For this review, take the finished solid that the model builds, in its own axes (mm). A direction names the side the tool comes from. Coordinates: 2 decimals unless noted, no trailing zeros. Loops run counter-clockwise (first coordinate to the right, second up) from the corner with the lowest first, then second, coordinate; pieces in that order, holes last. Notation, with made-up numbers: M -12.75,47 L 43.25,47 A16 cw 43.25,77 Z; hole C 2,49.25 d10. An arc over 180 degrees is marked long. Put each result on its own line as item: value.
```python
from build123d import *

# Parameters (mm, degrees)
F0_W     = 220
F0_H     = 25
F0_R     = 5
F1_DEPTH = 25
F2_DEPTH = 25


with BuildPart() as f1:
    # F0 (on Front) → F1 (new body)
    with BuildSketch(Plane.XZ):
        with Locations((103.33334, 12.5)):
            Rectangle(F0_W, F0_H)
        with Locations((3.33334, 12.5)):
            Circle(F0_R, mode=Mode.SUBTRACT)
        with Locations((203.33334, 12.5)):
            Circle(F0_R, mode=Mode.SUBTRACT)
        with Locations((3.33334, 12.5)):
            Circle(F0_R)
        with Locations((203.33334, 12.5)):
            Circle(F0_R)
    extrude(amount=F1_DEPTH)

    # F0 (on Front) → F2 (join)
    with BuildSketch(Plane.XZ):
        with Locations((3.33334, 12.5)):
            Circle(F0_R)
        with Locations((203.33334, 12.5)):
            Circle(F0_R)
    extrude(amount=-F2_DEPTH)


solid = f1.part
```
(1) Add section B-B (y = 12.5). Write out the cut boundary in (x, z).
Determined:
outline: C 3.33,12.5 d10; C 203.33,12.5 d10
(2) Draft analysis for pull direction X (two halves, no side actions). For faces 1 (the flat face through (213.333, -12, 12)), 2 (the cylindrical face through (198.34, 12.32, 12.72)), 3 (the flat face through (3, 25, 13)), 4 (the flat face through (-6.667, -12, 12)), state which applies: +X half, -X half, draft (parallel to the pull), parting line (faces both ways), or undercut.
Determined:
face 1: +X half
face 2: undercut
face 3: draft
face 4: -X half
(3) Add section A-A (z = 12.5). Write out the cut boundary in (x, y).
Determined:
outline: M -6.67,-25 L 213.33,-25 L 213.33,0 L 208.33,0 L 208.33,25 L 198.33,25 L 198.33,0 L 8.33,0 L 8.33,25 L -1.67,25 L -1.67,0 L -6.67,0 Z
(4) Wall thickness on line 1 along Y through (x, z) = (39, 2.75); line 2 along X through (y, z) = (16.5, 14.75); line 3 along X through (y, z) = (5.5, 8.75): over which ranges is each line inside the solid? List them lowest first. Write a range as [from, to].
Determined:
line 1: y = [-25, 0]
line 2: x = [-1.13, 7.8], [198.87, 207.8]
line 3: x = [0.03, 6.64], [200.03, 206.64]
(5) For pin 1 (10 mm diameter, centred on x = 147.5, z = 20.5, fed in from +Y); pin 2 (8 mm diameter, centred on y = 4.5, z = 18, fed in from -X); pin 3 (1.5 mm diameter, centred on x = 67.5, y = 1, fed in from +Z), all flat-tipped, find the tip position at first contact; note any pin that passes through.
Determined:
pin 1: stops at y = 0
pin 2: stops at x = -1.44
pin 3: passes through
(6) Add section C-C (x = 13). Write out the cut boundary in (y, z).
Determined:
outline: M -25,0 L 0,0 L 0,25 L -25,25 Z
(7) Tool access review of faces 5 (the flat face through (203, 25, 13)), 6 (the cylindrical face through (6.021, 12.325, 16.716)): name each direction out of +Z, -Z, +X, -X, +Y, -Y from which nothing blocks a thin tool from reaching the whole face with its end or side.
Determined:
face 5: +Z, -Z, +X, -X, +Y
face 6: +Y
